Design review of the part built by this model. Coordinates are the model's own, in mm. Face numbers are marked on the shaded views. Round coordinates to 2 decimals unless told otherwise and drop trailing zeros. Write each loop counter-clockwise with the first axis right and the second up, starting at its lowest first coordinate (ties: lowest second). Pieces come first, ordered by that corner, then holes.
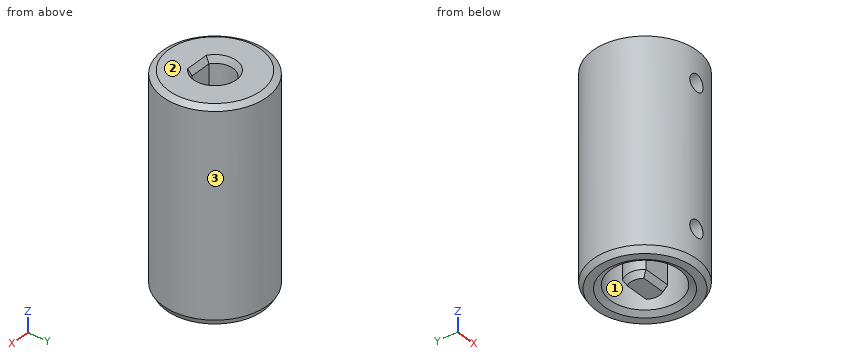
from build123d import *

# Parameters (mm, degrees)
OD_PROFILE_SKETCH_R                = 7.5
OD_BOSS_EXTRUDE_DEPTH              = 30
WHEEL_SHAFT_PROFILE_SKETCH_R       = 4.95
WHEEL_SHAFT_CUT_EXTRUDE_DEPTH      = 10
NEMA17_SHAFT_CUT_EXTRUDE_DEPTH     = 10
TAP_DRILL_FOR_M3X0_5_D             = 2.4
TAP_DRILL_FOR_M3X0_5_DEPTH         = 5.4
EDGE_CHAMFER_1MM_X_60_SIZE         = 0.5
EDGE_CHAMFER_1MM_X_60_SIZE2        = 0.866025404
EDGE_CHAMFER_1MM_X_60_PART_2_SIZE  = 0.5
EDGE_CHAMFER_1MM_X_60_PART_2_SIZE2 = 0.866025404
EDGE_CHAMFER_1MM_X_60_PART_3_SIZE  = 0.5
EDGE_CHAMFER_1MM_X_60_PART_3_SIZE2 = 0.866025404
EDGE_CHAMFER_1MM_X_60_PART_4_SIZE  = 0.5
EDGE_CHAMFER_1MM_X_60_PART_4_SIZE2 = 0.866025404
EDGE_CHAMFER_1MM_X_60_PART_5_SIZE  = 0.5
EDGE_CHAMFER_1MM_X_60_PART_5_SIZE2 = 0.866025404


with BuildPart() as part:
    # OD Profile Sketch → OD Boss-Extrude (new body)
    with BuildSketch(Plane.XY):
        Circle(OD_PROFILE_SKETCH_R)
    extrude(amount=OD_BOSS_EXTRUDE_DEPTH)

    # Wheel Shaft Profile Sketch → Wheel Shaft Cut-Extrude (cut)
    with BuildSketch(Plane.XY):
        Circle(WHEEL_SHAFT_PROFILE_SKETCH_R)
        with BuildLine():
            Line((1.967231557, -1.7), (-1.967231557, -1.7))
            ThreePointArc((-1.967231557, -1.7), (-2.6, 0), (-1.967231557, 1.7))
            Line((-1.967231557, 1.7), (1.967231557, 1.7))
            ThreePointArc((1.967231557, 1.7), (2.6, 0), (1.967231557, -1.7))
        make_face(mode=Mode.SUBTRACT)
    extrude(amount=WHEEL_SHAFT_CUT_EXTRUDE_DEPTH, mode=Mode.SUBTRACT)

    # NEMA17 Shaft Profile Sketch → NEMA17 Shaft Cut-Extrude (cut)
    with BuildSketch(Plane.XY.offset(30)):
        with BuildLine():
            Line((-1.532970972, -2.1), (1.532970972, -2.1))
            ThreePointArc((1.532970972, -2.1), (0, 2.6), (-1.532970972, -2.1))
        make_face()
    extrude(amount=-NEMA17_SHAFT_CUT_EXTRUDE_DEPTH, mode=Mode.SUBTRACT)

    # Tap Drill for M3x0.5
    with Locations(Plane(origin=(0, -7.5, 0), x_dir=(-1, 0, 0), z_dir=(0, -1, 0))):
        with Locations((0, -25), (0, -5)):
            Hole(TAP_DRILL_FOR_M3X0_5_D / 2, depth=TAP_DRILL_FOR_M3X0_5_DEPTH)

    # Edge Chamfer (1mm x 60)
    edge_chamfer_1mm_x_60_edges = [part.edges().sort_by_distance(p)[0] for p in [
        (-7.5, 0, 0),
    ]]
    edge_chamfer_1mm_x_60_side = [part.faces().sort_by_distance(p)[0] for p in [
        (-7.287867966, 0, 0),
    ]]
    chamfer(edge_chamfer_1mm_x_60_edges, length=EDGE_CHAMFER_1MM_X_60_SIZE, length2=EDGE_CHAMFER_1MM_X_60_SIZE2, reference=edge_chamfer_1mm_x_60_side[0])

    # Edge Chamfer (1mm x 60) part 2
    edge_chamfer_1mm_x_60_part_2_edges = [part.edges().sort_by_distance(p)[0] for p in [
        (0, 2.6, 30),
        (0, -2.1, 30),
    ]]
    edge_chamfer_1mm_x_60_part_2_side = [part.faces().sort_by_distance(p)[0] for p in [
        (-7.287867966, 0, 30),
    ]]
    chamfer(edge_chamfer_1mm_x_60_part_2_edges, length=EDGE_CHAMFER_1MM_X_60_PART_2_SIZE, length2=EDGE_CHAMFER_1MM_X_60_PART_2_SIZE2, reference=edge_chamfer_1mm_x_60_part_2_side[0])

    # Edge Chamfer (1mm x 60) part 3
    edge_chamfer_1mm_x_60_part_3_edges = [part.edges().sort_by_distance(p)[0] for p in [
        (-7.5, 0, 30),
    ]]
    edge_chamfer_1mm_x_60_part_3_side = [part.faces().sort_by_distance(p)[0] for p in [
        (-7.5, 0, 15),
    ]]
    chamfer(edge_chamfer_1mm_x_60_part_3_edges, length=EDGE_CHAMFER_1MM_X_60_PART_3_SIZE, length2=EDGE_CHAMFER_1MM_X_60_PART_3_SIZE2, reference=edge_chamfer_1mm_x_60_part_3_side[0])

    # Edge Chamfer (1mm x 60) part 4
    edge_chamfer_1mm_x_60_part_4_edges = [part.edges().sort_by_distance(p)[0] for p in [
        (2.6, 0, 0),
        (0, 1.7, 0),
        (-2.6, 0, 0),
        (0, -1.7, 0),
    ]]
    edge_chamfer_1mm_x_60_part_4_side = [part.faces().sort_by_distance(p)[0] for p in [
        (0, 0, 0),
    ]]
    chamfer(edge_chamfer_1mm_x_60_part_4_edges, length=EDGE_CHAMFER_1MM_X_60_PART_4_SIZE, length2=EDGE_CHAMFER_1MM_X_60_PART_4_SIZE2, reference=edge_chamfer_1mm_x_60_part_4_side[0])

    # Edge Chamfer (1mm x 60) part 5
    edge_chamfer_1mm_x_60_part_5_edges = [part.edges().sort_by_distance(p)[0] for p in [
        (-4.95, 0, 0),
    ]]
    edge_chamfer_1mm_x_60_part_5_side = [part.faces().sort_by_distance(p)[0] for p in [
        (-4.95, 0, 5),
    ]]
    chamfer(edge_chamfer_1mm_x_60_part_5_edges, length=EDGE_CHAMFER_1MM_X_60_PART_5_SIZE, length2=EDGE_CHAMFER_1MM_X_60_PART_5_SIZE2, reference=edge_chamfer_1mm_x_60_part_5_side[0])


solid = part.part
1) For line 1 along Z through (x, y) = (0, -6.2); line 2 along Z through (x, y) = (0, -5.4); line 3 along X through (y, z) = (-1.25, 2), list the stretches that pass through material, from the lowest coordinate up.
2) Add section B-B on z = 2.5. State the section outline as (x, y) points.
3) For P1, Ø1, axis at x = -3, z = 4.5, coming from the +Y side; P2, Ø1.2, axis at x = 1, z = 6, coming from the -Y side; P3, Ø5, axis at y = -6, z = 20, coming from the +X side, all flat-tipped, find the tip position at first contact; note any pin that passes through.
4) Add section D-D on z = 20.5. State the section outline as (x, y) points.
5) Add section A-A on x = 0. Count the separate pieces of the cut face and the enclosed holes in it, and give its area (3 significant figures).
6) Add section C-C on y = 0. State the section outline as (x, z) points.
7) The part is to be moulded in two halves that separate along X. For the marked faces 1, 2 and 3, say which applies: pulls with the +X half, pulls with the -X half, needs draft (parallel to the pull), parting line crosses it, or undercut.
Computed:
1. line 1: z = 0 to 3.8, 6.2 to 23.8, 26.2 to 30
1. line 2: z = 0.24 to 3.8, 6.2 to 23.8, 26.2 to 30
1. line 3: x = -7.4 to -4.79, -2.28 to 2.28, 4.79 to 7.4
2. outline: circle Ø15 at (0, 0); (-1.97, -1.7) - (1.97, -1.7) arc R2.6 ccw to (1.97, 1.7) - (-1.97, 1.7) arc R2.6 ccw to start; hole circle Ø9.9 at (0, 0)
3. P1: stops at y = 7.07
3. P2: stops at y = -7.49
3. P3: stops at x = 6.63
4. outline: circle Ø15 at (0, 0); hole (-1.53, -2.1) - (1.53, -2.1) arc R2.6 ccw (long way) to start
5. separate pieces: 3
5. enclosed holes: 0
5. area: 317 mm2
6. outline: (-7.5, 0.87) - (-7, 0) - (-5.82, 0) - (-4.95, 0.5) - (-4.95, 10) - (-2.6, 10) - (-2.6, 0.87) - (-2.1, 0) - (2.1, 0) - (2.6, 0.87) - (2.6, 10) - (4.95, 10) - (4.95, 0.5) - (5.82, 0) - (7, 0) - (7.5, 0.87) - (7.5, 29.5) - (6.63, 30) - (3.1, 30) - (2.6, 29.13) - (2.6, 20) - (-2.6, 20) - (-2.6, 29.13) - (-3.1, 30) - (-6.63, 30) - (-7.5, 29.5) - close
7. face 1: undercut
7. face 2: needs draft
7. face 3: parting line crosses it
